from build123d import *

# Parameters (mm, degrees)
SKETCH1_R                = 3.937
BOSS_EXTRUDE2_DEPTH      = 19.05
BOSS_EXTRUDE3_DEPTH      = 9.525
BOSS_EXTRUDE3_DEPTH_BACK = 28.575
SKETCH3_R                = 3.175


with BuildPart() as part:
    # Sketch1 → Boss-Extrude2 (new body)
    with BuildSketch(Plane.XY):
        with Locations(Location((0, 0, 0), (0, 0, 180))):
            Circle(SKETCH1_R)
    extrude(amount=BOSS_EXTRUDE2_DEPTH)

    # Sketch3 → Boss-Extrude3 (add, two sides: drawn at the far end of the back side and taken through both)
    with BuildSketch(Plane.XY.offset(19.05).offset(-BOSS_EXTRUDE3_DEPTH_BACK)):
        Circle(SKETCH3_R)
    extrude(amount=BOSS_EXTRUDE3_DEPTH + BOSS_EXTRUDE3_DEPTH_BACK)


solid = part.part
Could you check a few things on this model? Use its own coordinates, in mm. A direction names the side the tool comes from. Give positions to 0.01 mm unless a question says otherwise; leave off trailing zeros. Write each loop counter-clockwise with the first axis right and the second up, starting at its lowest first coordinate (ties: lowest second). Pieces come first, ordered by that corner, then holes. Notation, with made-up numbers: (78, 65.5) -> (112, 65.5) arc R32 cw to (112, 99.5) -> close; hole circle Ø1 at (-30.75, -38.5). An arc over 180 degrees is marked (long way). Answer as CSV lines item,"result". Start each with the question number.
(1) If we section it at A-A, the plane y = 0: Write out the boundary of the cut face in (x, z) (3 decimals), and give its area (3 significant figures).
(2) Which directions (+Z, -Z, +X, -X, +Y, -Y) give clear straight access to the entire face, cutting with the end or side of a thin tool? Please do faces 1 (the face through (0, 0, 28.575)), 2 (the face through (3, -2, 19.05)), 3 (the face through (-0.69, -3.1, -4.83)).
(3) I'm going to push flat-ended pins straight in: pin 1 Ø1 at (y, z) = (1.5, 14.5) entering from +X; pin 2 Ø3 at (y, z) = (-1.5, 21) entering from +X (3 decimals). Where does each tip first touch, or does it pass through?
(4) Please list where these lines run through material, in increasing order: line 1 (Z direction, x = -0.25, y = 3.25); line 2 (Y direction, x = 0.25, z = 5.5); line 3 (Y direction, x = -2.25, z = 22.5).
(5) If we section it at C-C, the plane z = 21.5: Write out the boundary of the cut face in (x, y) (3 decimals), and give its area (3 significant figures).
Answer list:
1,outline,"(-3.937, 0) -> (-3.175, 0) -> (-3.175, -9.525) -> (3.175, -9.525) -> (3.175, 0) -> (3.937, 0) -> (3.937, 19.05) -> (3.175, 19.05) -> (3.175, 28.575) -> (-3.175, 28.575) -> (-3.175, 19.05) -> (-3.937, 19.05) -> close"
1,area,"271 mm^2"
2,face 1,"+Z, +X, -X, +Y, -Y"
2,face 2,"+Z"
2,face 3,"-Z"
3,pin 1,"x = 3.81"
3,pin 2,"x = 3.175"
4,line 1,"0 to 19.05"
4,line 2,"-3.93 to 3.93"
4,line 3,"-2.24 to 2.24"
5,outline,"circle Ø6.35 at (0, 0)"
5,area,"31.7 mm^2"
